Verification items for the finished model (mm, model axes). A direction names the side the tool comes from. Round coordinates to 2 decimals unless told otherwise and drop trailing zeros. Order: outer loops, then holes, each group sorted by start corner. A loop starts at its lowest first (then second) coordinate and runs counter-clockwise, first axis right, second up. Notation, with made-up numbers: M 10.5,-0.5 L 16.5,-0.5 A29 cw 16.5,30.5 Z; hole C -5.5,-30 d3. An arc over 180 degrees is marked long. Answer as a JSON object with one key per item and string values. Group by question number.
Autodesk Inventor part; units mm, degrees
ref_plane "YZ Plane" through (0, 0, 0) normal (1, 0, 0) x (0, 1, 0)
ref_plane "XZ Plane" through (0, 0, 0) normal (0, 1, 0) x (-1, 0, 0)
ref_plane "XY Plane" through (0, 0, 0) normal (0, 0, 1) x (1, 0, 0)
sketch "Sketch1" plane through (0, 0, 0) normal (0, 1, 0) x (-1, 0, 0)
  line L0 (80, -141.4) -> (0, -141.4)
  line L1 (0, -141.4) -> (0, 0)
  line L2 (0, 0) -> (34.0381, 0)
  line L3 (34.0381, 0) -> (80, -45.9619)
  line L4 (80, -45.9619) -> (80, -141.4)
  dimension "d0" = 80
  dimension "d1" = 141.4
  dimension "d7" = 135
  dimension "d8" = 65
extrude "Extrusion1" add sketch "Sketch1" along normal blind 4
sketch "Sketch2" plane through (0, 4, 0) normal (0, 1, 0) x (1, 0, 0)
  line L0 (0, 0) -> (0, 141.4)
  line L1 (0, 0) -> (5, 0)
  line L2 (5, 0) -> (5, 141.4)
  line L3 (5, 141.4) -> (0, 141.4)
  line L4 (0, 141.4) -> (0, 0)
  point P0 (0, 141.4)
  dimension "d4" = 5
extrude "Extrusion2" add sketch "Sketch2" against normal blind 2
sketch "Sketch3" plane through (0, 4, 0) normal (0, 1, 0) x (1, 0, 0)
  line L0 (-34.0381, 0) -> (5, 0)
  line L1 (-29.7954, 0) -> (-35.4523, 5.6569)
  line L2 (-80, 45.9619) -> (-34.0381, 0)
  line L3 (-29.7954, 0) -> (-25.5528, 0)
  line L4 (-25.5528, 0) -> (-33.331, 7.7782)
  line L5 (-33.331, 7.7782) -> (-35.4523, 5.6569)
  line L6 (-77, 136.4) -> (-74, 136.4)
  line L7 (-74, 136.4) -> (-74, 141.4)
  line L8 (-74, 141.4) -> (-77, 141.4)
  line L9 (-77, 141.4) -> (-77, 136.4)
  line L10 (-80, 141.4) -> (-80, 45.9619)
  line L11 (5, 141.4) -> (-80, 141.4)
  point P0 (0, 0)
  dimension "d9" = 8
  dimension "d10" = 3
  dimension "d15" = 3
  dimension "d16" = 5
  dimension "d17" = 3
extrude "Extrusion3" add sketch "Sketch3" along normal blind 5
properties part number "side_wall"
Q1. Cross-section at A-A, the plane y = 6.25. Record the cut outline in (x, z), then the cut area to 3 significant figures.
Q2. Gauge pin test, flat ends, axial feed: pin 1 Ø1.5 at (y, z) = (5, -91) entering from +X; pin 2 Ø2.5 at (y, z) = (7, -138.5) entering from -X; pin 3 Ø2.5 at (x, z) = (3.5, -57) entering from -Y; pin 4 Ø3.5 at (x, y) = (-75, 7.5) entering from +Z. Record the tip position at first contact, or that the pin passes through.
Q3. Cross-section at B-B, the plane z = -54.5. Record the cut outline in (x, y).
Q4. Cross-section at C-C, the plane x = -7.5. Record the cut outline in (y, z), then the cut area to 3 significant figures.
Q5. Thickness scan on line 1 (Y direction, x = -25, z = -18.5); line 2 (X direction, y = 0.5, z = -117); line 3 (X direction, y = 2.5, z = -32.5). Record the ranges inside material, lowest first. Write a range as from..to.
Q6. Tool access check on faces 1 (the face through (-32.584, 6.465, -2.789)), 2 (the face through (2, 2, -72)), 3 (the face through (-29.387, 6.465, -3.835)). Record the directions out of +Z, -Z, +X, -X, +Y, -Y that give a thin tool (end or side, any length) a straight path to the whole face; none if there is none.
Q7. Cross-section at D-D, the plane x = -27. Record the cut outline in (y, z), then the cut area to 3 significant figures.
Conclusion:
{
 "1": {"outline": "M -77,-141.4 L -74,-141.4 L -74,-136.4 L -77,-136.4 Z; M -35.45,-5.66 L -33.33,-7.78 L -25.55,0 L -29.8,0 Z", "area": "43.5 mm2"},
 "2": {"pin 1": "through", "pin 2": "x = -77", "pin 3": "y = 2", "pin 4": "z = -136.4"},
 "3": {"outline": "M -80,0 L 0,0 L 0,2 L 5,2 L 5,4 L -80,4 Z"},
 "4": {"outline": "M 0,-141.4 L 4,-141.4 L 4,0 L 0,0 Z", "area": "566 mm2"},
 "5": {"line 1": "0..4", "line 2": "-80..0", "line 3": "-66.54..5"},
 "6": {"face 1": "+Z, -X, +Y", "face 2": "+Z, -Z, +X, -Y", "face 3": "-Z, +X, +Y"},
 "7": {"outline": "M 0,-141.4 L 4,-141.4 L 4,-1.45 L 9,-1.45 L 9,0 L 0,0 Z", "area": "573 mm2"}
}
